```python
from build123d import *

# Parameters (mm, degrees)
F0_W     = 139.7
F0_H     = 88.9
F1_DEPTH = 1219.2
F2_W     = 88.9
F2_H     = 139.7
F3_DEPTH = 38.1
F4_R     = 4.7625
F5_DEPTH = 25.4


with BuildPart() as f1:
    # F0 (on Top) → F1 (new body, symmetric)
    with BuildSketch(Plane.XY):
        Rectangle(F0_W, F0_H)
    extrude(amount=F1_DEPTH, both=True)

    # F2 (on face) → F3 (cut)
    with BuildSketch(Plane.YZ.offset(69.85)):
        with Locations((0, 996.95)):
            Rectangle(F2_W, F2_H)
        with Locations((0, -57.15)):
            Rectangle(F2_W, F2_H)
    extrude(amount=-F3_DEPTH, mode=Mode.SUBTRACT)

    # F4 (on face) → F5 (cut)
    with BuildSketch(Plane(origin=(-69.85, 0, 0), x_dir=(0, -1, 0), z_dir=(-1, 0, 0))):
        with Locations((0, -558.8)):
            Circle(F4_R)
        with Locations((0, 431.8)):
            Circle(F4_R)
        with Locations((0, 1143)):
            Circle(F4_R)
    extrude(amount=-F5_DEPTH, mode=Mode.SUBTRACT)


solid = f1.part
```
The model under review builds one solid part; all positions refer to its coordinate system, in mm. A direction names the side the tool comes from. Give positions to 0.01 mm unless a question says otherwise; leave off trailing zeros. Loops run counter-clockwise (first coordinate to the right, second up) from the corner with the lowest first, then second, coordinate; pieces in that order, holes last. Notation, with made-up numbers: (57.5, -34) - (91.5, -34) arc R20 cw to (91.5, -24) - close; hole circle Ø4 at (66, 21). An arc over 180 degrees is marked (long way). Answer as a JSON object with one key per item and string values.
Q1. Insertion check: pin 1 (5 mm diameter, centred on y = 2, z = -557.5, fed in from -X); pin 2 (3 mm diameter, centred on y = 2, z = 430, fed in from -X). Each pin has a flat end and moves straight along its axis. Give the tip position at first contact, or say it passes through.
Worked out:
{"pin 1": "stops at x = -69.85", "pin 2": "stops at x = -44.45"}
Q2. Add section B-B on z = -45.5. State the section outline as (x, y) points, plus the area to 3 significant figures.
Worked out:
{"outline": "(-69.85, -44.45) - (31.75, -44.45) - (31.75, 44.45) - (-69.85, 44.45) - close", "area": "9,030 mm^2"}
Q3. For faces 4 (the flat face through (31.75, -1, 998)), 5 (the flat face through (-1, 1, 1219.2)), list the 3-axis set-ups (+Z, -Z, +X, -X, +Y, -Y) from which the entire face can be reached by the end or side of a thin tool; tool diameter is ignored.
Worked out:
{"face 4": "+X, +Y, -Y", "face 5": "+Z, +X, -X, +Y, -Y"}
Q4. Add section A-A on y = 30.5. State the section outline as (x, z) points, plus the area to 3 significant figures.
Worked out:
{"outline": "(-69.85, -1219.2) - (69.85, -1219.2) - (69.85, -127) - (31.75, -127) - (31.75, 12.7) - (69.85, 12.7) - (69.85, 927.1) - (31.75, 927.1) - (31.75, 1066.8) - (69.85, 1066.8) - (69.85, 1219.2) - (-69.85, 1219.2) - close", "area": "330,000 mm^2"}
Q5. To check wall thickness, follow line 1 along Z through (x, y) = (50.5, 19); line 2 along Z through (x, y) = (-50.25, 0); line 3 along Y through (x, z) = (-55, 1143). State the ranges of each line that lie inside material, in increasing order.
Worked out:
{"line 1": "z = -1219.2 to -127, 12.7 to 927.1, 1066.8 to 1219.2", "line 2": "z = -1219.2 to -563.56, -554.04 to 427.04, 436.56 to 1138.24, 1147.76 to 1219.2", "line 3": "y = -44.45 to -4.76, 4.76 to 44.45"}
Q6. Mouldability with a two-part tool opening along Z and no side actions: class faces 1 (the flat face through (51, -1, -127)), 2 (the flat face through (-1, 1, -1219.2)), 3 (the flat face through (-69.85, -1, 17)) as +Z half, -Z half, draft (parallel to the pull), parting line (faces both ways), or undercut.
Worked out:
{"face 1": "undercut", "face 2": "-Z half", "face 3": "draft"}
